Geometry check sheet. Reference: the model listing, model coordinates, mm. Face numbers are marked on the shaded views. A direction names the side the tool comes from. Round coordinates to 2 decimals unless told otherwise and drop trailing zeros. Loops run counter-clockwise (first coordinate to the right, second up) from the corner with the lowest first, then second, coordinate; pieces in that order, holes last. Notation, with made-up numbers: M 40.5,54.25 L 78.5,54.25 A9 ccw 78.5,61.25 Z; hole C -6.75,61.25 d8. An arc over 180 degrees is marked long. Write item = value, one per line.
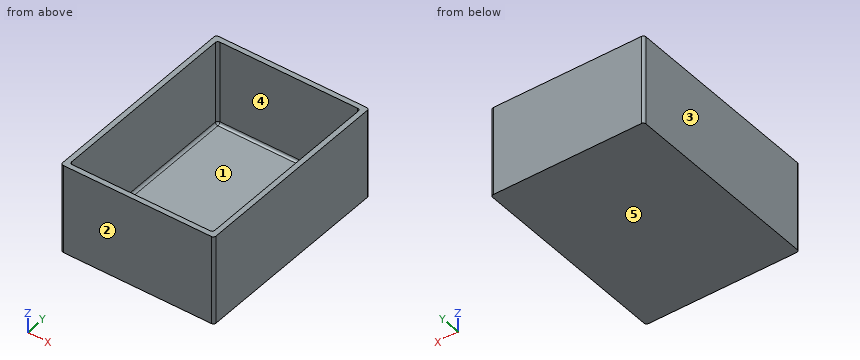
from build123d import *

# Parameters (mm, degrees)
F0_W     = 76.2
F0_H     = 101.6
F1_DEPTH = 44.45
F2_T     = -2.54
F3_R     = 1.27
F4_R     = 1.27


with BuildPart() as f1:
    # F0 (on Top) → F1 (new body)
    with BuildSketch(Plane.XY):
        with Locations((38.1, 50.8)):
            Rectangle(F0_W, F0_H)
    extrude(amount=F1_DEPTH)

    # F2
    f2_openings = [f1.faces().sort_by_distance(p)[0] for p in [
        (38.1, 50.8, 44.45),
    ]]
    offset(amount=F2_T, openings=f2_openings)

    # F3
    f3_edges = [f1.edges().sort_by_distance(p)[0] for p in [
        (2.54, 2.54, 23.495),
        (2.54, 99.06, 23.495),
        (73.66, 2.54, 23.495),
        (73.66, 99.06, 23.495),
        (0, 0, 22.225),
        (0, 101.6, 22.225),
        (76.2, 0, 22.225),
        (76.2, 101.6, 22.225),
    ]]
    fillet(f3_edges, radius=F3_R)

    # F4
    f4_edges = [f1.edges().sort_by_distance(p)[0] for p in [
        (2.54, 50.8, 2.54),
        (2.911974, 98.688026, 2.54),
        (2.911974, 2.911974, 2.54),
        (38.1, 99.06, 2.54),
        (38.1, 2.54, 2.54),
        (73.288026, 98.688026, 2.54),
        (73.288026, 2.911974, 2.54),
        (73.66, 50.8, 2.54),
    ]]
    fillet(f4_edges, radius=F4_R)


solid = f1.part
(1) Sectioned sample at A-A on z = 33.5. Record the cut outline in (x, y), then the cut area to 3 significant figures.
Result set:
outline = M 0,1.27 A1.27 ccw 1.27,0 L 74.93,0 A1.27 ccw 76.2,1.27 L 76.2,100.33 A1.27 ccw 74.93,101.6 L 1.27,101.6 A1.27 ccw 0,100.33 Z; hole M 2.54,3.81 A1.27 ccw 3.81,2.54 L 72.39,2.54 A1.27 ccw 73.66,3.81 L 73.66,97.79 A1.27 ccw 72.39,99.06 L 3.81,99.06 A1.27 ccw 2.54,97.79 Z
area = 877 mm2
(2) Release check for a two-part mould opening along X. For the marked faces 3, 4 and 5 record: released by +X, released by -X, zero draft, split by the parting line, or undercut.
Result set:
face_3 = released by -X
face_4 = undercut
face_5 = zero draft
(3) Tool access check on the marked faces 1 and 2. Record the directions out of +Z, -Z, +X, -X, +Y, -Y that give a thin tool (end or side, any length) a straight path to the whole face; none if there is none.
Result set:
face_1 = +Z
face_2 = +Z, -Z, +X, -X, -Y
(4) Material ranges on line 1 along X through (y, z) = (92.5, 14); line 2 along Y through (x, z) = (43, 18); line 3 along Z through (x, y) = (66, 49), recorded low to high. Write a range as from..to.
Result set:
line_1 = 0..2.54, 73.66..76.2
line_2 = 0..2.54, 99.06..101.6
line_3 = 0..2.54
(5) Sectioned sample at B-B on y = 14.5. Record the cut outline in (x, z).
Result set:
outline = M 0,0 L 76.2,0 L 76.2,44.45 L 73.66,44.45 L 73.66,3.81 A1.27 cw 72.39,2.54 L 3.81,2.54 A1.27 cw 2.54,3.81 L 2.54,44.45 L 0,44.45 Z
(6) Sectioned sample at C-C on x = 30.5. Record the cut outline in (y, z), then the cut area to 3 significant figures.
Result set:
outline = M 0,0 L 101.6,0 L 101.6,44.45 L 99.06,44.45 L 99.06,3.81 A1.27 cw 97.79,2.54 L 3.81,2.54 A1.27 cw 2.54,3.81 L 2.54,44.45 L 0,44.45 Z
area = 472 mm2
